```python
from build123d import *

# Parameters (mm, degrees)
SKETCH1_R                = 1.6
BOSS_EXTRUDE1_DEPTH      = 11.15
SKETCH2_W                = 82
SKETCH2_H                = 0.6
CUT_EXTRUDE1_DEPTH       = 8
CUT_EXTRUDE2_DEPTH       = 46.2
CUT_EXTRUDE3_DEPTH       = 40.2
CUT_EXTRUDE5_DEPTH       = 39.2
BOSS_EXTRUDE2_DEPTH      = 32.2
CHAMFER3_SIZE            = 1.1
CHAMFER4_SIZE            = 1.1
CUT_EXTRUDE12_DEPTH      = 1
CUT_EXTRUDE12_DEPTH_BACK = 83
FILLET3_R                = 15
SKETCH14_R               = 1.6
CUT_EXTRUDE14_DEPTH      = 12.1500001
BOSS_EXTRUDE3_DEPTH      = 3.5
SKETCH8_W                = 82
SKETCH8_H                = 0.6
CUT_EXTRUDE16_DEPTH      = 4.15
CUT_EXTRUDE17_DEPTH      = 2.4
CHAMFER5_SIZE            = 0.5


with BuildPart() as part:
    # Sketch1 → Boss-Extrude1 (new body)
    with BuildSketch(Plane.XY):
        with BuildLine():
            Line((0, -35.2), (82, -35.2))
            Line((82, -35.2), (82, 8.75))
            ThreePointArc((82, 8.75), (81.165254326, 10.765254326), (79.15, 11.6))
            Line((79.15, 11.6), (2.85, 11.6))
            ThreePointArc((2.85, 11.6), (0.834745674, 10.765254326), (0, 8.75))
            Line((0, 8.75), (0, -35.2))
        make_face()
        with Locations((4, 8.939640599)):
            Circle(SKETCH1_R, mode=Mode.SUBTRACT)
        with Locations((78, 8.939640599)):
            Circle(SKETCH1_R, mode=Mode.SUBTRACT)
    extrude(amount=BOSS_EXTRUDE1_DEPTH)

    # Sketch2 → Cut-Extrude1 (cut)
    with BuildSketch(Plane(origin=(0, 0, 0), x_dir=(-1, 0, 0), z_dir=(0, 0, -1))):
        with Locations((-41, -34.9)):
            Rectangle(SKETCH2_W, SKETCH2_H)
    cut_extrude1 = extrude(amount=-CUT_EXTRUDE1_DEPTH, mode=Mode.SUBTRACT)

    # Sketch3 → Cut-Extrude2 (cut)
    with BuildSketch(Plane.XZ.offset(34.6)):
        with BuildLine():
            Line((25.85, 4), (25.85, 0))
            Line((25.85, 0), (29.15, 0))
            Line((29.15, 0), (29.15, 4))
            ThreePointArc((29.15, 4), (27.5, 5.65), (25.85, 4))
        make_face()
        with BuildLine():
            ThreePointArc((14.15, 4), (12.5, 5.65), (10.85, 4))
            Line((10.85, 4), (10.85, 0))
            Line((10.85, 0), (14.15, 0))
            Line((14.15, 0), (14.15, 4))
        make_face()
        with BuildLine():
            ThreePointArc((23.25, 4), (20, 7.25), (16.75, 4))
            Line((16.75, 4), (16.75, 0))
            Line((16.75, 0), (23.25, 0))
            Line((23.25, 0), (23.25, 4))
        make_face()
    cut_extrude2 = extrude(amount=-CUT_EXTRUDE2_DEPTH, mode=Mode.SUBTRACT)

    # Sketch4 → Cut-Extrude3 (cut)
    with BuildSketch(Plane(origin=(0, 11.6, 0), x_dir=(1, 0, 0), z_dir=(0, 1, 0))):
        with BuildLine():
            Line((9.25, -4), (9.25, 0))
            Line((9.25, 0), (15.75, 0))
            Line((15.75, 0), (15.75, -4))
            ThreePointArc((15.75, -4), (12.5, -7.25), (9.25, -4))
        make_face()
        with BuildLine():
            Line((24.25, -4), (24.25, 0))
            Line((24.25, 0), (30.75, 0))
            Line((30.75, 0), (30.75, -4))
            ThreePointArc((30.75, -4), (27.5, -7.25), (24.25, -4))
        make_face()
    cut_extrude3 = extrude(amount=-CUT_EXTRUDE3_DEPTH, mode=Mode.SUBTRACT)

    # Sketch6 → Cut-Extrude5 (cut)
    with BuildSketch(Plane(origin=(0, 11.6, 0), x_dir=(1, 0, 0), z_dir=(0, 1, 0))):
        with BuildLine():
            Line((15.75, -4), (15.75, 0))
            Line((15.75, 0), (15.75, 0.65176216))
            Line((15.75, 0.65176216), (0, 0.65176216))
            Line((0, 0.65176216), (0, -7.25))
            Line((0, -7.25), (12.5, -7.25))
            ThreePointArc((12.5, -7.25), (14.798097039, -6.298097039), (15.75, -4))
        make_face()
        with BuildLine():
            Line((24.25, 0), (24.25, -4))
            ThreePointArc((24.25, -4), (25.201902961, -6.298097039), (27.5, -7.25))
            Line((27.5, -7.25), (41, -7.25))
            Line((41, -7.25), (41, 0))
            Line((41, 0), (24.25, 0))
        make_face()
    cut_extrude5 = extrude(amount=-CUT_EXTRUDE5_DEPTH, mode=Mode.SUBTRACT)

    # Mirror1: Cut-Extrude1, Cut-Extrude2, Cut-Extrude3, Cut-Extrude5 across plane
    add(cut_extrude1.mirror(Plane.ZY.offset(-41)), mode=Mode.SUBTRACT)
    add(cut_extrude2.mirror(Plane.ZY.offset(-41)), mode=Mode.SUBTRACT)
    add(cut_extrude3.mirror(Plane.ZY.offset(-41)), mode=Mode.SUBTRACT)
    add(cut_extrude5.mirror(Plane.ZY.offset(-41)), mode=Mode.SUBTRACT)

    # Sketch12 → Boss-Extrude2 (add)
    with BuildSketch(Plane(origin=(0, 11.6, 0), x_dir=(1, 0, 0), z_dir=(0, 1, 0))):
        with BuildLine():
            Line((16.75, -4), (16.75, 0))
            Line((16.75, 0), (18, 0))
            Line((18, 0), (18.11, -3.084631222))
            ThreePointArc((18.11, -3.084631222), (20, -6.1), (21.89, -3.084631222))
            Line((21.89, -3.084631222), (22, 0))
            Line((22, 0), (23.25, 0))
            Line((23.25, 0), (23.25, -4))
            ThreePointArc((23.25, -4), (20, -7.25), (16.75, -4))
        make_face()
        with BuildLine():
            Line((58.75, -4), (58.75, 0))
            Line((58.75, 0), (60.05, 0))
            Line((60.05, 0), (60.155, -3.106425717))
            ThreePointArc((60.155, -3.106425717), (62, -6.05), (63.845, -3.106425717))
            Line((63.845, -3.106425717), (63.95, 0))
            Line((63.95, 0), (65.25, 0))
            Line((65.25, 0), (65.25, -4))
            ThreePointArc((65.25, -4), (62, -7.25), (58.75, -4))
        make_face()
    extrude(amount=-BOSS_EXTRUDE2_DEPTH)

    # Chamfer3
    chamfer3_edges = [part.edges().sort_by_distance(p)[0] for p in [
        (65.25, -20.6, 2),
        (58.75, -20.6, 2),
        (62, -20.6, 7.25),
    ]]
    chamfer(chamfer3_edges, length=CHAMFER3_SIZE)

    # Chamfer4
    chamfer4_edges = [part.edges().sort_by_distance(p)[0] for p in [
        (23.25, -20.6, 2),
        (16.75, -20.6, 2),
        (20, -20.6, 7.25),
    ]]
    chamfer(chamfer4_edges, length=CHAMFER4_SIZE)

    # Sketch9 → Cut-Extrude12 (cut, two sides)
    with BuildSketch(Plane.ZY) as cut_extrude12_sk:
        Polygon((-106.219800457, 11.6), (0, 11.6), (7.25, 11.6), (0, 2.4), (-65.744961499, -81.028089075), (-260.411588221, -166.089763625), (-300.886427179, -73.46167455), align=None)
    extrude(amount=CUT_EXTRUDE12_DEPTH, mode=Mode.SUBTRACT)
    extrude(cut_extrude12_sk.sketch, amount=-CUT_EXTRUDE12_DEPTH_BACK, mode=Mode.SUBTRACT)

    # Fillet3
    fillet3_edges = [part.edges().sort_by_distance(p)[0] for p in [
        (16.875, 2.4, 0),
        (23.125, 2.4, 0),
        (58.9, 2.4, 0),
        (65.1, 2.4, 0),
    ]]
    fillet(fillet3_edges, radius=FILLET3_R)

    # Sketch14 → Cut-Extrude14 (cut, through all)
    with BuildSketch(Plane.XY.offset(11.15)):
        with Locations((4, -19.400359401)):
            Circle(SKETCH14_R)
    cut_extrude14 = extrude(amount=-CUT_EXTRUDE14_DEPTH, mode=Mode.SUBTRACT)

    # Mirror3: Cut-Extrude14 across plane
    add(cut_extrude14.mirror(Plane.ZY.offset(-41)), mode=Mode.SUBTRACT)

    # Sketch18 → Boss-Extrude3 (add)
    with BuildSketch(Plane(origin=(0, -27.6, 0), x_dir=(1, 0, 0), z_dir=(0, 1, 0))):
        with BuildLine():
            Line((14.15, 0), (14.15, -1.2))
            ThreePointArc((14.15, -1.2), (15.321790212, -2.38754845), (15.75, -4))
            Line((15.75, -4), (15.75, 0))
            Line((15.75, 0), (14.15, 0))
        make_face()
        with BuildLine():
            Line((10.85, -1.2), (10.85, 0))
            Line((10.85, 0), (9.25, 0))
            Line((9.25, 0), (9.25, -4))
            ThreePointArc((9.25, -4), (9.678209788, -2.38754845), (10.85, -1.2))
        make_face()
        with BuildLine():
            Line((29.15, 0), (29.15, -1.2))
            ThreePointArc((29.15, -1.2), (30.321790212, -2.38754845), (30.75, -4))
            Line((30.75, -4), (30.75, 0))
            Line((30.75, 0), (29.15, 0))
        make_face()
        with BuildLine():
            Line((25.85, -1.2), (25.85, 0))
            Line((25.85, 0), (24.25, 0))
            Line((24.25, 0), (24.25, -4))
            ThreePointArc((24.25, -4), (24.678209788, -2.38754845), (25.85, -1.2))
        make_face()
    boss_extrude3 = extrude(amount=-BOSS_EXTRUDE3_DEPTH)

    # Mirror5: Boss-Extrude3 across plane
    add(boss_extrude3.mirror(Plane.ZY.offset(-41)))

    # Sketch8 → Cut-Extrude16 (cut, through all)
    with BuildSketch(Plane(origin=(0, 0, 8), x_dir=(-1, 0, 0), z_dir=(0, 0, -1))):
        with Locations((-41, -34.9)):
            Rectangle(SKETCH8_W, SKETCH8_H)
    extrude(amount=-CUT_EXTRUDE16_DEPTH, mode=Mode.SUBTRACT)

    # Sketch20 → Cut-Extrude17 (cut)
    with BuildSketch(Plane(origin=(0, 0, 7.25), x_dir=(-1, 0, 0), z_dir=(0, 0, -1))):
        Polygon((-80.9, 12.288272161), (-75.1, 12.288272161), (-75.1, 7.265324819), (-78, 5.591009038), (-84.071495483, 9.096388589), align=None)
        Polygon((-75.1, -21.074675181), (-75.1, -17.72604362), (-78, -16.051727839), (-80.9, -17.72604362), (-80.9, -21.074675181), (-78, -22.748990962), align=None)
    cut_extrude17 = extrude(amount=-CUT_EXTRUDE17_DEPTH, mode=Mode.SUBTRACT)

    # Mirror7: Cut-Extrude17 across plane
    add(cut_extrude17.mirror(Plane.ZY.offset(-41)), mode=Mode.SUBTRACT)

    # Chamfer5
    chamfer5_edges = [part.edges().sort_by_distance(p)[0] for p in [
        (2.4, 8.939640599, 11.15),
        (76.4, 8.939640599, 11.15),
        (2.4, -19.400359401, 11.15),
        (79.6, -19.400359401, 11.15),
    ]]
    chamfer(chamfer5_edges, length=CHAMFER5_SIZE)


solid = part.part
```
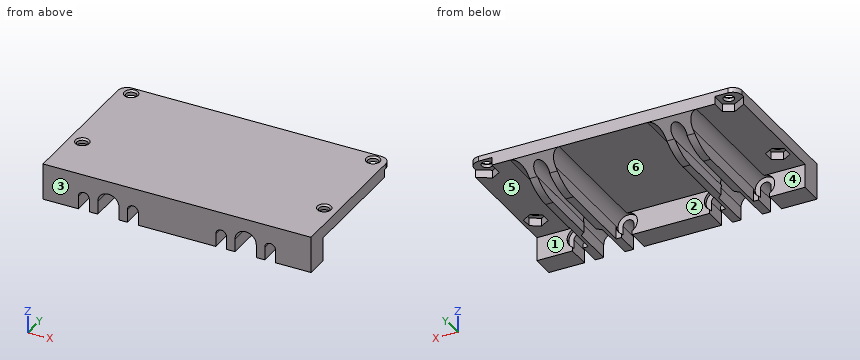
Geometry check sheet. Reference: the model listing, model coordinates, mm. Face numbers are marked on the shaded views. A direction names the side the tool comes from. Coordinates: 2 decimals unless noted, no trailing zeros. Loops run counter-clockwise (first coordinate to the right, second up) from the corner with the lowest first, then second, coordinate; pieces in that order, holes last. Notation, with made-up numbers: (-34.5, 47) - (24.5, 47) arc R4 cw to (24.5, 51) - close; hole circle Ø3 at (38.5, -33.5). An arc over 180 degrees is marked (long way). One line per item, written item: value. Start each with the question number.
(1) Tool access check on the marked faces 3, 4, 5 and 6. Record the directions out of +Z, -Z, +X, -X, +Y, -Y that give a thin tool (end or side, any length) a straight path to the whole face; none if there is none.
(2) Mould release check, pull along X, two halves, no side actions. Record for the marked faces 1 and 2: released by +X, released by -X, zero draft, split by the parting line, or undercut.
(3) Material ranges on line 1 (X direction, y = -9.5, z = 4); line 2 (Y direction, x = 4, z = 10.25); line 3 (X direction, y = -11.5, z = 3), recorded low to high. Write a range as [from, to].
(4) Depth check by flat-ended pin: P1, Ø1, axis at x = 21.5, z = 5, coming from the +Y side; P2, Ø1.2, axis at y = -1.5, z = 2, coming from the +X side; P3, Ø5, axis at x = 2.5, y = 8, coming from the -Z side. Enter the tip coordinate at first touch or a pass-through.
(5) Cross-section at C-C on x = 20. Enter the section's corners in (y, z), plus the area to 3 significant figures.
(6) Cross-section at A-A on y = -31. Enter the section's corners in (x, z).
(7) Cross-section at B-B on x = 62. Enter the section's corners in (y, z), plus the area to 3 significant figures.
Results below:
1. face 3: +Z, -Z, +X, -X, -Y
1. face 4: -Z, -X, +Y
1. face 5: -Z, +X, +Y
1. face 6: -Z, +Y
2. face 1: zero draft
2. face 2: undercut
3. line 1: x = [15.75, 17.9], [22.1, 24.25], [57.75, 59.95], [64.05, 66.25]
3. line 2: y = [-34.6, -21], [-17.8, 7.34], [10.54, 11.6]
3. line 3: x = [15.75, 18.11], [21.89, 24.25], [57.75, 60.15], [63.85, 66.25]
4. P1: stops at y = 9.38
4. P2: stops at x = 66.25
4. P3: stops at z = 7.25
5. outline: (-34.6, 7.25) - (-21.7, 7.25) - (-20.6, 6.15) - (-20.6, 6.1) - (10.14, 6.1) - (11.6, 7.25) - (11.6, 11.15) - (-34.6, 11.15) - close
5. area: 217 mm2
6. outline: (0, 0) - (10.85, 0) - (10.85, 4) arc R1.65 cw to (14.15, 4) - (14.15, 0) - (16.75, 0) - (16.75, 4) arc R3.25 cw to (23.25, 4) - (23.25, 0) - (25.85, 0) - (25.85, 4) arc R1.65 cw to (29.15, 4) - (29.15, 0) - (52.85, 0) - (52.85, 4) arc R1.65 cw to (56.15, 4) - (56.15, 0) - (58.75, 0) - (58.75, 4) arc R3.25 cw to (65.25, 4) - (65.25, 0) - (67.85, 0) - (67.85, 4) arc R1.65 cw to (71.15, 4) - (71.15, 0) - (82, 0) - (82, 11.15) - (0, 11.15) - close
7. outline: (-34.6, 7.25) - (-21.7, 7.25) - (-20.6, 6.15) - (-20.6, 6.05) - (10.08, 6.05) - (11.6, 7.25) - (11.6, 11.15) - (-34.6, 11.15) - close
7. area: 219 mm2
